Can you work these out from the model? Positions are in its coordinate system, mm. Face numbers are marked on the shaded views. Round coordinates to 2 decimals unless told otherwise and drop trailing zeros. Order: outer loops, then holes, each group sorted by start corner. A loop starts at its lowest first (then second) coordinate and runs counter-clockwise, first axis right, second up. Notation, with made-up numbers: M 81,-17.5 L 97,-17.5 A31 ccw 97,13.5 Z; hole C -6,-39 d11. An arc over 180 degrees is marked long. Answer as a JSON object with one key per item and string values. Group by question number.
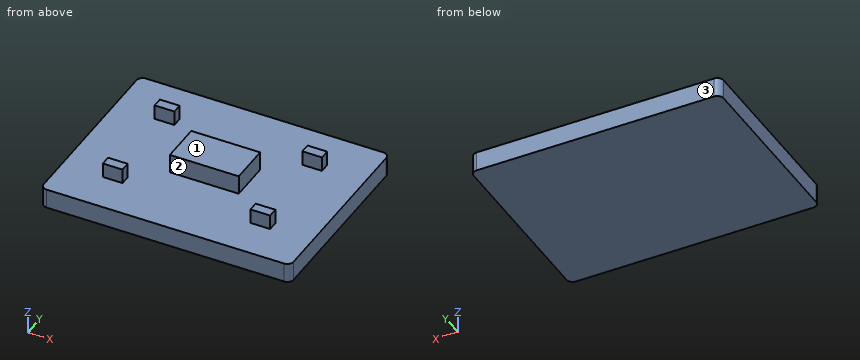
from build123d import *

# Parameters (mm, degrees)
PCB_DEPTH   = 1.6
IC_SK2_W    = 5.6
IC_SK2_H    = 3.3
IC_DEPTH    = 1.55
PARTS_SK3_W = 1.6
PARTS_SK3_H = 0.8
PARTS_DEPTH = 1.2


with BuildPart() as part:
    # PCB_Sk1 → PCB (new body)
    with BuildSketch(Plane.XY.offset(-2)):
        with BuildLine():
            Line((19.35, 3.35), (38.65, 3.35))
            ThreePointArc((38.65, 3.35), (39.003553391, 3.496446609), (39.15, 3.85))
            Line((39.15, 3.85), (39.15, 18.15))
            ThreePointArc((39.15, 18.15), (39.003553391, 18.503553391), (38.65, 18.65))
            Line((38.65, 18.65), (19.35, 18.65))
            ThreePointArc((19.35, 18.65), (18.996446609, 18.503553391), (18.85, 18.15))
            Line((18.85, 18.15), (18.85, 3.85))
            ThreePointArc((18.85, 3.85), (18.996446609, 3.496446609), (19.35, 3.35))
        make_face()
    extrude(amount=-PCB_DEPTH)

    # IC_Sk2 → IC (add)
    with BuildSketch(Plane.XY.offset(-2)):
        with Locations((29, 11)):
            Rectangle(IC_SK2_W, IC_SK2_H)
    extrude(amount=IC_DEPTH)

    # Parts_Sk3 → Parts (add)
    with BuildSketch(Plane.XY.offset(-2)):
        with Locations((23, 7)):
            Rectangle(PARTS_SK3_W, PARTS_SK3_H)
        with Locations((23, 15)):
            Rectangle(PARTS_SK3_W, PARTS_SK3_H)
        with Locations((35, 7)):
            Rectangle(PARTS_SK3_W, PARTS_SK3_H)
        with Locations((35, 15)):
            Rectangle(PARTS_SK3_W, PARTS_SK3_H)
    extrude(amount=PARTS_DEPTH)


solid = part.part
Item 1: Suppose I cut it at B-B, the plane x = 23.5. Write out the boundary of the cut face in (y, z), and give its area (3 significant figures).
Item 2: Suppose I cut it at D-D, the plane x = 27.5. Write out the boundary of the cut face in (y, z).
Item 3: I need wall thicknesses on line 1 (Y direction, x = 22.25, z = -1.5); line 2 (Y direction, x = 29.75, z = -0.8); line 3 (Z direction, x = 35.5, y = 17.25). Which ranges of each line are inside material? Lowest first, please.
Item 4: Suppose I cut it at A-A, the plane z = -1.5. Write out the boundary of the cut face in (x, y), and give its area (3 significant figures).
Item 5: I'm going to push flat-ended pins straight in: pin 1 Ø0.6 at (y, z) = (7, -1.5) entering from -X; pin 2 Ø1.2 at (y, z) = (11, -1) entering from -X; pin 3 Ø0.8 at (x, z) = (29, -1.5) entering from +Y. Where does each tip first touch, or does it pass through?
Item 6: If we mould it in two halves opening along Y, with no side actions, what happens to the marked faces 1, 2 and 3? For each: +Y half, -Y half, draft (parallel to the pull), parting line (faces both ways), or undercut.
Item 7: Suppose I cut it at C-C, the plane y = 15. Write out the boundary of the cut face in (x, z).
Computed:
{
 "1": {"outline": "M 3.35,-3.6 L 18.65,-3.6 L 18.65,-2 L 15.4,-2 L 15.4,-0.8 L 14.6,-0.8 L 14.6,-2 L 7.4,-2 L 7.4,-0.8 L 6.6,-0.8 L 6.6,-2 L 3.35,-2 Z", "area": "26.4 mm^2"},
 "2": {"outline": "M 3.35,-3.6 L 18.65,-3.6 L 18.65,-2 L 12.65,-2 L 12.65,-0.45 L 9.35,-0.45 L 9.35,-2 L 3.35,-2 Z"},
 "3": {"line 1": "y = 6.6 to 7.4, 14.6 to 15.4", "line 2": "y = 9.35 to 12.65", "line 3": "z = -3.6 to -2"},
 "4": {"outline": "M 22.2,6.6 L 23.8,6.6 L 23.8,7.4 L 22.2,7.4 Z; M 22.2,14.6 L 23.8,14.6 L 23.8,15.4 L 22.2,15.4 Z; M 26.2,9.35 L 31.8,9.35 L 31.8,12.65 L 26.2,12.65 Z; M 34.2,6.6 L 35.8,6.6 L 35.8,7.4 L 34.2,7.4 Z; M 34.2,14.6 L 35.8,14.6 L 35.8,15.4 L 34.2,15.4 Z", "area": "23.6 mm^2"},
 "5": {"pin 1": "stops at x = 22.2", "pin 2": "stops at x = 26.2", "pin 3": "stops at y = 12.65"},
 "6": {"face 1": "draft", "face 2": "-Y half", "face 3": "+Y half"},
 "7": {"outline": "M 18.85,-3.6 L 39.15,-3.6 L 39.15,-2 L 35.8,-2 L 35.8,-0.8 L 34.2,-0.8 L 34.2,-2 L 23.8,-2 L 23.8,-0.8 L 22.2,-0.8 L 22.2,-2 L 18.85,-2 Z"}
}
